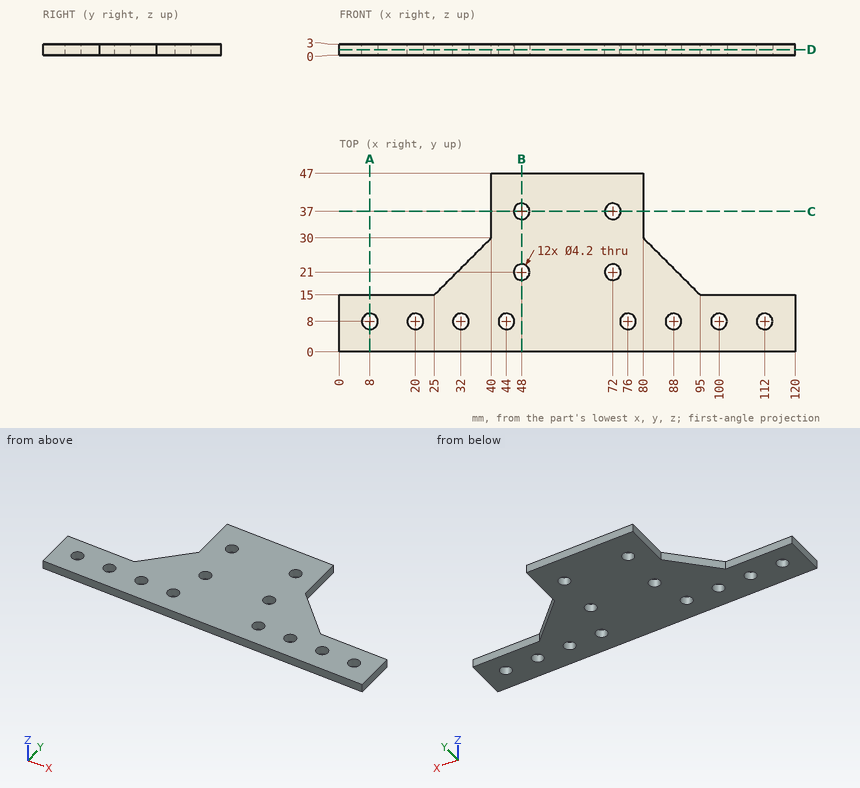
Source: three-view drawing plus pictorial views. Frame: mm from the lowest corner of the part. Round coordinates to 2 decimals unless told otherwise and drop trailing zeros. Write each loop counter-clockwise with the first axis right and the second up, starting at its lowest first coordinate (ties: lowest second). Pieces come first, ordered by that corner, then holes. Notation, with made-up numbers: M 19,75.5 L 63,75.5 A30 cw 63,99.5 Z; hole C 44.25,-26.5 d4. An arc over 180 degrees is marked long. One line per item, written item: value. Start each with the question number.
Item 1: Pin query (flat end, axial travel): pin 1 (12 mm diameter, centred on x = 81, y = 37.5, fed in from +Z); pin 2 (1.5 mm diameter, centred on x = 37, z = 2.5, fed in from +Y); pin 3 (1.5 mm diameter, centred on y = 38.5, z = 1.5, fed in from +X); pin 4 (0.9 mm diameter, centred on x = 108, z = 2, fed in from +Y). Return the tip coordinate at first contact, or that it passes through.
Item 2: Section query A-A (x = 8). Return the cut outline in (y, z), plus the area to 3 significant figures.
Item 3: Ray query, L1, parallel to Y at x = 72, z = 2.35; L2, parallel to Y at x = 44, z = 0.9; L3, parallel to Y at x = 8, z = 2. Return the intervals inside material, ascending. Write a range as from..to.
Item 4: Section query C-C (y = 37). Return the cut outline in (x, z).
Item 5: Section query D-D (z = 1.5). State how many separate pieces and enclosed holes the cut face has, plus the area to 3 significant figures.
Item 6: Section query B-B (x = 48). Return the cut outline in (y, z), plus the area to 3 significant figures.
Result set:
1. pin 1: stops at z = 3
1. pin 2: stops at y = 27.75
1. pin 3: stops at x = 80
1. pin 4: stops at y = 15
2. outline: M 0,0 L 5.9,0 L 5.9,3 L 0,3 Z; M 10.1,0 L 15,0 L 15,3 L 10.1,3 Z
2. area: 32.4 mm²
3. L1: y = 0..18.9, 23.1..34.9, 39.1..47
3. L2: y = 0..5.9, 10.1..47
3. L3: y = 0..5.9, 10.1..15
4. outline: M 40,0 L 45.9,0 L 45.9,3 L 40,3 Z; M 50.1,0 L 69.9,0 L 69.9,3 L 50.1,3 Z; M 74.1,0 L 80,0 L 80,3 L 74.1,3 Z
5. separate pieces: 1
5. enclosed holes: 12
5. area: 3,140 mm²
6. outline: M 0,0 L 18.9,0 L 18.9,3 L 0,3 Z; M 23.1,0 L 34.9,0 L 34.9,3 L 23.1,3 Z; M 39.1,0 L 47,0 L 47,3 L 39.1,3 Z
6. area: 116 mm²
